Geometry: final body of the model. Coordinates: model frame, mm. A direction names the side the tool comes from. Round coordinates to 2 decimals unless told otherwise and drop trailing zeros. Loops run counter-clockwise (first coordinate to the right, second up) from the corner with the lowest first, then second, coordinate; pieces in that order, holes last. Notation, with made-up numbers: (24.25, -12) -> (28.25, -12) arc R17 ccw to (28.25, 14) -> close; hole circle Ø7 at (85.5, 54.5). An arc over 180 degrees is marked (long way). Answer in a Markdown table with one row per item.
```python
from build123d import *

# Parameters (mm, degrees)
DODANIE_WYCI_GNI_CIE1_DEPTH      = 17
ZAOKR_GLENIE1_R                  = 2
DODANIE_WYCI_GNI_CIE2_DEPTH      = 2
ZAOKR_GLENIE2_R                  = 1
ZAOKR_GLENIE3_R                  = 1
WYTNIJ_WYCI_GNI_CIE1_DEPTH       = 32.35628887
WYTNIJ_WYCI_GNI_CIE1_DEPTH_BACK  = 32.35628887
SZKIC4_R                         = 2.1
DODANIE_WYCI_GNI_CIE3_DEPTH      = 6
DODANIE_WYCI_GNI_CIE3_DEPTH_BACK = 6
SZKIC9_R                         = 2.1
SZKIC8_R                         = 1.9
WYTNIJ_WYCI_GNI_CIE3_DEPTH       = 10.5
ZAOKR_GLENIE5_R                  = 2
WYTNIJ_WYCI_GNI_CIE4_DEPTH       = 6.5
SZKIC12_R                        = 0.75
WYTNIJ_WYCI_GNI_CIE5_DEPTH       = 6.5


with BuildPart() as part:
    # Szkic1 → Dodanie-wyciągnięcie1 (new body)
    with BuildSketch(Plane.XY):
        Polygon((1.783068787, -4.564092652), (-0.653727134, 7.430712848), (-12.25993137, 11.317788426), (-21.429339686, 3.210058505), (-18.992543765, -8.784746995), (-7.386339528, -12.671822573), align=None)
    extrude(amount=DODANIE_WYCI_GNI_CIE1_DEPTH)

    # Zaokrąglenie1
    zaokr_glenie1_edges = [part.edges().sort_by_distance(p)[0] for p in [
        (-7.386339528, -12.671822573, 8.5),
        (-18.992543765, -8.784746995, 8.5),
        (-21.429339686, 3.210058505, 8.5),
        (-12.25993137, 11.317788426, 8.5),
        (-0.653727134, 7.430712848, 8.5),
        (1.783068787, -4.564092652, 8.5),
    ]]
    fillet(zaokr_glenie1_edges, radius=ZAOKR_GLENIE1_R)

    # Szkic3 → Dodanie-wyciągnięcie2 (add)
    with BuildSketch(Plane.XY.offset(17)):
        Polygon((-0.091452095, 7.927884965), (-12.409357535, 12.053318952), (-22.141040889, 3.448416913), (-19.554818803, -9.281919113), (-7.236913363, -13.407353099), (2.494769991, -4.80245106), align=None)
    extrude(amount=-DODANIE_WYCI_GNI_CIE2_DEPTH)

    # Zaokrąglenie2
    zaokr_glenie2_edges = [part.edges().sort_by_distance(p)[0] for p in [
        (-6.456829252, 9.374250637, 0),
        (-2.80163537, -8.617957613, 0),
        (-13.189441647, -10.728284784, 0),
        (-20.210941725, -2.787344245, 0),
        (-16.844635528, 7.263923465, 0),
        (0.564670827, 1.433310098, 0),
        (-12.198333493, 11.014581025, 0),
        (-21.135955436, 3.111800131, 0),
        (-18.760757392, -8.579797968, 0),
        (-7.447937406, -12.368615173, 0),
        (1.489684537, -4.465834278, 0),
        (-0.885513507, 7.225763821, 0),
    ]]
    fillet(zaokr_glenie2_edges, radius=ZAOKR_GLENIE2_R)

    # Zaokrąglenie3
    zaokr_glenie3_edges = [part.edges().sort_by_distance(p)[0] for p in [
        (1.201658948, 1.562716953, 17),
        (-6.250404815, 9.990601959, 17),
        (-17.275199212, 7.750867932, 17),
        (-20.847929846, -2.9167511, 17),
        (-13.395866083, -11.344636106, 17),
        (-2.371071686, -9.10490208, 17),
    ]]
    fillet(zaokr_glenie3_edges, radius=ZAOKR_GLENIE3_R)

    # Szkic4 → Wytnij-wyciągnięcie1 (cut, two sides: drawn at the far end of the back side and taken through both)
    with BuildSketch(Plane(origin=(-0.257260592, 1.266331223, 0), x_dir=(0.9799817241599056, 0.19908746899937949, 0), z_dir=(-0.19908746899937946, 0.9799817241599055, 0)).offset(-WYTNIJ_WYCI_GNI_CIE1_DEPTH_BACK)):
        with Locations(Location((-9.76127883, -5.05, 0), (0, 0, 241.563109851))):
            Circle(SZKIC4_R)
    extrude(amount=WYTNIJ_WYCI_GNI_CIE1_DEPTH + WYTNIJ_WYCI_GNI_CIE1_DEPTH_BACK, mode=Mode.SUBTRACT)

    # Szkic9 → Dodanie-wyciągnięcie3 (add, two sides: drawn at the far end of the back side and taken through both)
    with BuildSketch(Plane(origin=(-0.257260592, 1.266331223, 0), x_dir=(0.9799817241599056, 0.19908746899937949, 0), z_dir=(-0.19908746899937946, 0.9799817241599055, 0)).offset(-DODANIE_WYCI_GNI_CIE3_DEPTH_BACK)):
        with Locations(Location((-9.76127883, -5.05, 0), (0, 0, 180))):
            Circle(SZKIC9_R)
    extrude(amount=DODANIE_WYCI_GNI_CIE3_DEPTH + DODANIE_WYCI_GNI_CIE3_DEPTH_BACK)

    # Szkic8 → Wytnij-wyciągnięcie3 (cut)
    with BuildSketch(Plane.XY.offset(17)):
        with Locations((-9.823135449, -0.677017074)):
            Circle(SZKIC8_R)
    extrude(amount=-WYTNIJ_WYCI_GNI_CIE3_DEPTH, mode=Mode.SUBTRACT)

    # Zaokrąglenie5
    zaokr_glenie5_edges = [part.edges().sort_by_distance(p)[0] for p in [
        (-11.723135449, -0.677017074, 17),
    ]]
    fillet(zaokr_glenie5_edges, radius=ZAOKR_GLENIE5_R)

    # Szkic11 → Wytnij-wyciągnięcie4 (cut)
    with BuildSketch(Plane(origin=(0, 0, 0), x_dir=(-1, 0, 0), z_dir=(0, 0, -1))):
        Polygon((13.831970706, 1.978023394), (12.478175917, -4.68585233), (5.814300193, -3.332057541), (7.168094982, 3.331818183), align=None)
    extrude(amount=-WYTNIJ_WYCI_GNI_CIE4_DEPTH, mode=Mode.SUBTRACT)

    # Szkic12 → Wytnij-wyciągnięcie5 (cut)
    with BuildSketch(Plane(origin=(0, 0, 0), x_dir=(-1, 0, 0), z_dir=(0, 0, -1))):
        with Locations((13.831970706, 1.978023394)):
            Circle(SZKIC12_R)
        with Locations((12.478175917, -4.68585233)):
            Circle(SZKIC12_R)
        with Locations((5.814300193, -3.332057541)):
            Circle(SZKIC12_R)
        with Locations((7.168094982, 3.331818183)):
            Circle(SZKIC12_R)
    extrude(amount=-WYTNIJ_WYCI_GNI_CIE5_DEPTH, mode=Mode.SUBTRACT)


solid = part.part
```
Item 1: Cut plane C-C (z = 5.75). Output: boundary loops of the cut face in (x, y).
Answer:
| item | result |
|---|---|
| outline | (-21.2, 2.08) -> (-19.22, -7.65) arc R2 ccw to (-17.9, -9.15) -> (-9.55, -11.95) -> (-10.57, -6.95) -> (-6.69, -6.16) -> (-5.67, -11.16) -> (0.92, -5.33) arc R2 ccw to (1.55, -3.43) -> (-0.42, 6.3) arc R2 ccw to (-1.75, 7.8) -> (-10.09, 10.59) -> (-9.08, 5.6) -> (-12.96, 4.81) -> (-13.97, 9.8) -> (-20.56, 3.97) arc R2 ccw to start; hole (-13.68, 1.24) -> (-12.63, -3.95) arc R0.75 ccw (long way) to (-11.74, -4.54) -> (-6.55, -3.48) arc R0.75 ccw (long way) to (-5.96, -2.6) -> (-7.02, 2.6) arc R0.75 ccw (long way) to (-7.9, 3.18) -> (-13.1, 2.13) arc R0.75 ccw (long way) to start |
Item 2: Line query: probe 1 along Z at (x, y) = (-9.75, -7); probe 2 along X at (y, z) = (-2.25, 8); probe 3 along Y at (x, z) = (-11.5, 10.25). Output: solid intervals per line, ascending. Write a range as [from, to].
Answer:
| item | result |
|---|---|
| probe 1 | z = [0, 3.32], [6.78, 17] |
| probe 2 | x = [-20.32, -10.89], [-8.76, 1.31] |
| probe 3 | y = [-11.29, -1.57], [0.22, 11.03] |
Item 3: Draft query along X for faces 1 (the face through (-17.15, 7.48, 16.7)), 2 (the face through (0.9, 1.6, 16.7)), 3 (the face through (-10.464, 2.662, 3.204)). Return one class per face: pulls with the +X half, pulls with the -X half, needs draft (parallel to the pull), parting line crosses it, or undercut.
Answer:
| item | result |
|---|---|
| face 1 | pulls with the -X half |
| face 2 | pulls with the +X half |
| face 3 | undercut |
Item 4: Reachability of faces 4 (the face through (-0.876, 7.215, 8.098)), 5 (the face through (-8.6, -6.55, 5.08)), 6 (the face through (-21.13, 3.13, 8.1)), 7 (the face through (-13.255, -10.706, 7.902)) from +Z, -Z, +X, -X, +Y, -Y: full face, straight path, thin tool, end or side. Return the list, or none.
Answer:
| item | result |
|---|---|
| face 4 | -Z, +X, +Y |
| face 5 | none |
| face 6 | -Z, -X |
| face 7 | -Z, -X, -Y |
Item 5: Cut plane D-D (z = 4). Output: boundary loops of the cut face in (x, y).
Answer:
| item | result |
|---|---|
| outline | (-21.2, 2.08) -> (-19.22, -7.65) arc R2 ccw to (-17.9, -9.15) -> (-9.38, -12) -> (-10.41, -6.92) -> (-6.85, -6.19) -> (-5.81, -11.28) -> (0.92, -5.33) arc R2 ccw to (1.55, -3.43) -> (-0.42, 6.3) arc R2 ccw to (-1.75, 7.8) -> (-10.27, 10.65) -> (-9.24, 5.56) -> (-12.8, 4.84) -> (-13.83, 9.93) -> (-20.56, 3.97) arc R2 ccw to start; hole (-13.68, 1.24) -> (-12.63, -3.95) arc R0.75 ccw (long way) to (-11.74, -4.54) -> (-6.55, -3.48) arc R0.75 ccw (long way) to (-5.96, -2.6) -> (-7.02, 2.6) arc R0.75 ccw (long way) to (-7.9, 3.18) -> (-13.1, 2.13) arc R0.75 ccw (long way) to start |
Item 6: Cut plane B-B (z = 14). Output: boundary loops of the cut face in (x, y) (1 decimal).
Answer:
| item | result |
|---|---|
| outline | (-21.2, 2.1) -> (-19.2, -7.7) arc R2 ccw to (-17.9, -9.2) -> (-8.5, -12.3) arc R2 ccw to (-6.5, -11.9) -> (0.9, -5.3) arc R2 ccw to (1.6, -3.4) -> (-0.4, 6.3) arc R2 ccw to (-1.7, 7.8) -> (-11.2, 11) arc R2 ccw to (-13.1, 10.6) -> (-20.6, 4) arc R2 ccw to start; hole circle Ø3.8 at (-9.8, -0.7) |
Item 7: Pin query (flat end, axial travel): pin 1 Ø10 at (y, z) = (-10, 2.5) entering from +X; pin 2 Ø2 at (x, z) = (-4, 6.5) entering from +Y; pin 3 Ø5 at (x, z) = (-6, 12) entering from +Y. Return the tip coordinate at first contact, or that it passes through.
Answer:
| item | result |
|---|---|
| pin 1 | stops at x = 1.22 |
| pin 2 | stops at y = 8.89 |
| pin 3 | stops at y = 10.06 |
